Can you work these out from the model? Positions are in its coordinate system, mm. A direction names the side the tool comes from. Give positions to 0.01 mm unless a question says otherwise; leave off trailing zeros.
from build123d import *

# Parameters (mm, degrees)
BOSS_EXTRUDE2_DEPTH      = 52
FILLET2_R                = 1
CUT_EXTRUDE2_DEPTH       = 3
CUT_EXTRUDE2_DEPTH_BACK  = 6
SKETCH10_W               = 2.071027546
SKETCH10_H               = 17.5
SKETCH12_W               = 21
SKETCH12_H               = 29
BATTERY_DEPTH            = 0.4
SKETCH14_W               = 21.3
SKETCH14_H               = 1
BOSS_EXTRUDE4_DEPTH      = 7.999920354
FILLET5_R                = 1
SKETCH19_W               = 21.3
SKETCH19_H               = 1
BOSS_EXTRUDE5_DEPTH      = 2.6
SKETCH20_W               = 9.556221564
SKETCH20_H               = 2.6
CUT_EXTRUDE9_DEPTH       = 2.6
SKETCH21_W               = 21.3
SKETCH21_H               = 2.886084762
BOSS_EXTRUDE6_DEPTH      = 8
SKETCH23_W               = 24.481547991
SKETCH23_H               = 2.403526745
CUT_EXTRUDE10_DEPTH      = 2
SKETCH26_W               = 11.036128308
SKETCH26_H               = 2.126226966
CUT_EXTRUDE11_DEPTH      = 2
CUT_EXTRUDE12_DEPTH      = 2
CUT_EXTRUDE12_DEPTH_BACK = 11
SKETCH27_W               = 46
SKETCH27_H               = 2.33
CUT_EXTRUDE15_DEPTH      = 3
CUT_EXTRUDE15_DEPTH_BACK = 2
SKETCH30_W               = 16.027497941
SKETCH30_H               = 8.207966742
SKETCH32_W               = 21.3
SKETCH32_H               = 4.3
BOSS_EXTRUDE7_DEPTH      = 17
SKETCH33_W               = 15.5
SKETCH33_H               = 4.8
CUT_EXTRUDE16_DEPTH      = 17
CUT_EXTRUDE17_DEPTH      = 16
CUT_EXTRUDE17_DEPTH_BACK = 16
SKETCH34_W               = 15.546115034
SKETCH34_H               = 15
CHAMFER1_SIZE            = 2.050303842
CHAMFER1_SIZE_2          = 1
SKETCH36_W               = 1.919218309
SKETCH36_H               = 1.441495618
BOSS_EXTRUDE8_DEPTH      = 24
SKETCH37_W               = 15.546115034
SKETCH37_H               = 5.800639797
CUT_EXTRUDE18_DEPTH      = 3
SKETCH38_W               = 4.259754253
SKETCH38_H               = 3
BOSS_EXTRUDE9_DEPTH      = 7
FILLET6_R                = 2.5
BOSS_EXTRUDE10_DEPTH     = 18
SKETCH41_W               = 2.868853839
SKETCH41_H               = 1
SKETCH41_W_2             = 2.885031127
BOSS_EXTRUDE11_DEPTH     = 3
SKETCH42_W               = 6.004877842
SKETCH42_H               = 3.067097043
CUT_EXTRUDE19_DEPTH      = 7


with BuildPart() as part:
    # Sketch1 → Boss-Extrude2 (new body)
    with BuildSketch(Plane.XY):
        with BuildLine():
            Line((-4.570161627, 0), (-7.263800128, 0))
            add(Edge.make_bspline(
                [(0.042333709, 8.998333002), (-4.213116867, 8.648828695), (-5.985828681, 2.169241543), (-7.263800128, 0)],
                knots=[0, 0, 0, 0, 1, 1, 1, 1], degree=3))
            Line((0.042333709, 8.998333002), (0.742333709, 8.998333002))
            Line((0.742333709, 8.998333002), (0.742333709, 1))
            Line((0.742333709, 1), (22.042333709, 1))
            Line((22.042333709, 1), (22.042333709, 8.998333002))
            Line((22.042333709, 8.998333002), (23.042333709, 8.998333002))
            add(Edge.make_bspline(
                [(23.042333709, 8.998333002), (27.852391375, 8.27132168), (31.467788923, 0)],
                knots=[0, 0, 0, 1, 1, 1], degree=2))
            Line((31.467788923, 0), (26.875523276, 0))
            Line((26.875523276, 0), (22.86911945, 0))
            Line((22.86911945, 0), (0, 0))
            Line((0, 0), (-4.570161627, 0))
        make_face()
    extrude(amount=BOSS_EXTRUDE2_DEPTH)

    # Fillet2
    fillet2_edges = [part.edges().sort_by_distance(p)[0] for p in [
        (-7.263800128, 0, 26),
    ]]
    fillet(fillet2_edges, radius=FILLET2_R)

    # Sketch10 → Cut-Extrude2 (cut, two sides: drawn at the far end of the back side and taken through both)
    with BuildSketch(Plane(origin=(-4.432649633, 3.861619691, 0), x_dir=(0.6568701979277837, 0.7540036757697632, 0), z_dir=(-0.7540036757697632, 0.6568701979277837, 0)).offset(-CUT_EXTRUDE2_DEPTH_BACK)):
        with Locations((-0.442686988, -41.317163409)):
            Rectangle(SKETCH10_W, SKETCH10_H)
        with Locations((-0.442686988, -11.478878468)):
            Rectangle(SKETCH10_W, SKETCH10_H)
    extrude(amount=CUT_EXTRUDE2_DEPTH + CUT_EXTRUDE2_DEPTH_BACK, mode=Mode.SUBTRACT)

    # Sketch12 → Battery (cut)
    with BuildSketch(Plane(origin=(0, 1, 0), x_dir=(1, 0, 0), z_dir=(0, 1, 0))):
        with Locations((11.242333709, -36.5)):
            Rectangle(SKETCH12_W, SKETCH12_H)
    extrude(amount=-BATTERY_DEPTH, mode=Mode.SUBTRACT)

    # Sketch14 → Boss-Extrude4 (add)
    with BuildSketch(Plane(origin=(0, 1, 0), x_dir=(1, 0, 0), z_dir=(0, 1, 0))):
        with Locations((11.392333709, -51.5)):
            Rectangle(SKETCH14_W, SKETCH14_H)
    extrude(amount=BOSS_EXTRUDE4_DEPTH)

    # Fillet5
    fillet5_edges = [part.edges().sort_by_distance(p)[0] for p in [
        (31.467788923, 0, 26),
    ]]
    fillet(fillet5_edges, radius=FILLET5_R)

    # Sketch19 → Boss-Extrude5 (add)
    with BuildSketch(Plane(origin=(0, 0, 51), x_dir=(-1, 0, 0), z_dir=(0, 0, -1))):
        with Locations((-11.392333709, 5)):
            Rectangle(SKETCH19_W, SKETCH19_H)
    extrude(amount=BOSS_EXTRUDE5_DEPTH)

    # Sketch20 → Cut-Extrude9 (cut)
    with BuildSketch(Plane(origin=(0, 5.5, 0), x_dir=(1, 0, 0), z_dir=(0, 1, 0))):
        with Locations((10.971722634, -49.7)):
            Rectangle(SKETCH20_W, SKETCH20_H)
    extrude(amount=-CUT_EXTRUDE9_DEPTH, mode=Mode.SUBTRACT)

    # Sketch21 → Boss-Extrude6 (add)
    with BuildSketch(Plane(origin=(0, 1, 0), x_dir=(1, 0, 0), z_dir=(0, 1, 0))):
        with Locations((11.392333709, -18.443042381)):
            Rectangle(SKETCH21_W, SKETCH21_H)
    extrude(amount=BOSS_EXTRUDE6_DEPTH)

    # Sketch23 → Cut-Extrude10 (cut)
    with BuildSketch(Plane(origin=(0.742333709, 0, 0), x_dir=(0, 0, -1), z_dir=(1, 0, 0))):
        with Locations((-32.126858758, 6.701763373)):
            Rectangle(SKETCH23_W, SKETCH23_H)
    extrude(amount=-CUT_EXTRUDE10_DEPTH, mode=Mode.SUBTRACT)

    # Sketch26 → Cut-Extrude11 (cut)
    with BuildSketch(Plane(origin=(0, 0, 51), x_dir=(-1, 0, 0), z_dir=(0, 0, -1))):
        with Locations((-6.260397863, 7.936806871)):
            Rectangle(SKETCH26_W, SKETCH26_H)
    extrude(amount=-CUT_EXTRUDE11_DEPTH, mode=Mode.SUBTRACT)

    # Sketch27 → Cut-Extrude12 (cut, two sides: drawn at the far end of the back side and taken through both)
    with BuildSketch(Plane(origin=(15.71645511, 16.134429341, 0), x_dir=(0, 0, -1), z_dir=(0.6977674498915984, 0.7163243580053493, 0)).offset(-CUT_EXTRUDE12_DEPTH_BACK)):
        with Locations((-26, -18.013212029)):
            Rectangle(SKETCH27_W, SKETCH27_H)
    extrude(amount=CUT_EXTRUDE12_DEPTH + CUT_EXTRUDE12_DEPTH_BACK, mode=Mode.SUBTRACT)

    # Sketch30 → Cut-Extrude15 (cut, two sides: drawn at the far end of the back side and taken through both)
    with BuildSketch(Plane(origin=(-4.432649633, 3.861619691, 0), x_dir=(0.6568701979277837, 0.7540036757697632, 0), z_dir=(-0.7540036757697632, 0.6568701979277837, 0)).offset(-CUT_EXTRUDE15_DEPTH_BACK)):
        with Locations((1.087669114, -26.408883952)):
            Rectangle(SKETCH30_W, SKETCH30_H)
    extrude(amount=CUT_EXTRUDE15_DEPTH + CUT_EXTRUDE15_DEPTH_BACK, mode=Mode.SUBTRACT)

    # Sketch32 → Boss-Extrude7 (add)
    with BuildSketch(Plane(origin=(0, 0, 0), x_dir=(-1, 0, 0), z_dir=(0, 0, -1))):
        with Locations((-11.392333709, 3.15)):
            Rectangle(SKETCH32_W, SKETCH32_H)
    extrude(amount=-BOSS_EXTRUDE7_DEPTH)

    # Sketch33 → Cut-Extrude16 (cut)
    with BuildSketch(Plane(origin=(0, 0, 0), x_dir=(-1, 0, 0), z_dir=(0, 0, -1))):
        with Locations((-11.42347987, 2.9)):
            Rectangle(SKETCH33_W, SKETCH33_H)
    extrude(amount=-CUT_EXTRUDE16_DEPTH, mode=Mode.SUBTRACT)

    # Sketch34 → Cut-Extrude17 (cut, two sides: drawn at the far end of the back side and taken through both)
    with BuildSketch(Plane(origin=(0, 0.5, 0), x_dir=(1, 0, 0), z_dir=(0, 1, 0)).offset(-CUT_EXTRUDE17_DEPTH_BACK)):
        with Locations((11.400422353, -9.617701537)):
            Rectangle(SKETCH34_W, SKETCH34_H)
    extrude(amount=CUT_EXTRUDE17_DEPTH + CUT_EXTRUDE17_DEPTH_BACK, mode=Mode.SUBTRACT)

    # Chamfer1
    # the kernel refuses this chamfer: 2.050303842, 1 mm, written as the material it takes off along each edge
    with BuildSketch(Plane(origin=(19.17347987, 0.5, 2.117701537), x_dir=(0, 0.016923890849829, -0.9998567807033681), z_dir=(-1, 0, 0))) as chamfer1_piece_1:
        Polygon((CHAMFER1_SIZE * 0.999856780498, CHAMFER1_SIZE * 0.0169238908464), (-CHAMFER1_SIZE_2 * 0.0169238908498, CHAMFER1_SIZE_2 * 0.999856780703), (0, 0), align=None)
    extrude(amount=15.5, mode=Mode.SUBTRACT)

    # Sketch36 → Boss-Extrude8 (add)
    with BuildSketch(Plane(origin=(0.742333709, 0, 0), x_dir=(0, 0, -1), z_dir=(1, 0, 0))):
        with Locations((-0.959609155, 6.020747809)):
            Rectangle(SKETCH36_W, SKETCH36_H)
    extrude(amount=BOSS_EXTRUDE8_DEPTH)

    # Sketch37 → Cut-Extrude18 (cut)
    with BuildSketch(Plane(origin=(0, 0, 17.117701537), x_dir=(-1, 0, 0), z_dir=(0, 0, -1))):
        with Locations((-11.400422353, 4.08463089)):
            Rectangle(SKETCH37_W, SKETCH37_H)
    extrude(amount=-CUT_EXTRUDE18_DEPTH, mode=Mode.SUBTRACT)

    # Sketch38 → Boss-Extrude9 (add)
    with BuildSketch(Plane(origin=(0, 1.184310992, 0), x_dir=(1, 0, 0), z_dir=(0, 1, 0))):
        with Locations((11.677903031, -18.617701537)):
            Rectangle(SKETCH38_W, SKETCH38_H)
    extrude(amount=BOSS_EXTRUDE9_DEPTH)

    # Fillet6
    # the kernel refuses this fillet: 2.5 mm, written as the material it takes off along each edge
    with BuildSketch(Plane(origin=(14.862488739, 1.184310992, 17.117701537), x_dir=(0, -1, 0), z_dir=(-1, 0, 0))) as fillet6_piece_1_section:
        with BuildLine():
            CenterArc((2.5, 2.125785134), FILLET6_R, 180, 58.245844015)
            Line((0, 2.125785134), (-0.05, 2.125785134))
            Line((-0.05, 2.125785134), (-0.05, 0))
            Line((-0.05, 0), (0, -0.05))
            ThreePointArc((0, -0.05), (0.592155496, -0.05), (1.157997212, -0.042515703))
            Line((1.157997212, -0.042515703), (1.184310992, 0))
        make_face()
    fillet6_piece_1 = extrude(amount=11.235123902, mode=Mode.PRIVATE)
    fillet6_piece_1 = split(fillet6_piece_1, bisect_by=Plane(origin=(13.807780157, 0.878026012, 17.652561739), z_dir=(1, 0, 0)), keep=Keep.TOP, mode=Mode.PRIVATE)
    add(fillet6_piece_1, mode=Mode.SUBTRACT)
    with BuildSketch(Plane(origin=(9.548025904, 1.184310992, 17.117701537), x_dir=(0, -1, 0), z_dir=(-1, 0, 0))) as fillet6_piece_2:
        with BuildLine():
            CenterArc((2.5, 2.125785134), FILLET6_R, 180, 58.245844015)
            Line((0, 2.125785134), (-0.05, 2.125785134))
            Line((-0.05, 2.125785134), (-0.05, 0))
            Line((-0.05, 0), (0, -0.05))
            ThreePointArc((0, -0.05), (0.592155496, -0.05), (1.157997212, -0.042515703))
            Line((1.157997212, -0.042515703), (1.184310992, 0))
        make_face()
    extrude(amount=5.920661068, mode=Mode.SUBTRACT)
    with BuildSketch(Plane(origin=(19.17347987, 1.184310992, 17.117701537), x_dir=(0, -1, 0), z_dir=(-1, 0, 0))) as fillet6_piece_3:
        with BuildLine():
            CenterArc((2.5, 2.125785134), FILLET6_R, 180, 58.245844015)
            Line((0, 2.125785134), (-0.05, 2.125785134))
            Line((-0.05, 2.125785134), (-0.05, 0))
            Line((-0.05, 0), (0, -0.05))
            ThreePointArc((0, -0.05), (0.592155496, -0.05), (1.157997212, -0.042515703))
            Line((1.157997212, -0.042515703), (1.184310992, 0))
        make_face()
    extrude(amount=5.365699713, mode=Mode.SUBTRACT)
    with BuildSketch(Plane(origin=(19.17347987, 1.184310992, 17.117701537), x_dir=(0, -1, 0), z_dir=(-1, 0, 0))) as fillet6_piece_4_section:
        with BuildLine():
            CenterArc((2.5, 2.125785134), FILLET6_R, 180, 58.245844015)
            Line((0, 2.125785134), (-0.05, 2.125785134))
            Line((-0.05, 2.125785134), (-0.05, 0))
            Line((-0.05, 0), (0, -0.05))
            ThreePointArc((0, -0.05), (0.592155496, -0.05), (1.157997212, -0.042515703))
            Line((1.157997212, -0.042515703), (1.184310992, 0))
        make_face()
    fillet6_piece_4 = extrude(amount=10.680162547, mode=Mode.PRIVATE)
    fillet6_piece_4 = split(fillet6_piece_4, bisect_by=Plane(origin=(9.548025904, 0.878026012, 17.652561739), z_dir=(-1, 0, 0)), keep=Keep.TOP, mode=Mode.PRIVATE)
    add(fillet6_piece_4, mode=Mode.SUBTRACT)

    # Sketch40 → Boss-Extrude10 (add)
    with BuildSketch(Plane(origin=(3.67347987, 0, 0), x_dir=(0, 0, -1), z_dir=(1, 0, 0))):
        Polygon((-1.194674299, 0), (-2.117701537, 0), (-2.117701537, 0.29858263), (-1.194674299, 0.29858263), (-0.66544558, 0.29858263), (-0.66544558, 0), align=None)
    extrude(amount=BOSS_EXTRUDE10_DEPTH)

    # Sketch41 → Boss-Extrude11 (add)
    with BuildSketch(Plane.XY.offset(19.886084762)):
        with Locations((20.607906789, 5)):
            Rectangle(SKETCH41_W, SKETCH41_H)
        with Locations((2.184849273, 5)):
            Rectangle(SKETCH41_W_2, SKETCH41_H)
    extrude(amount=BOSS_EXTRUDE11_DEPTH)

    # Sketch42 → Cut-Extrude19 (cut)
    with BuildSketch(Plane(origin=(0, 9, 0), x_dir=(1, 0, 0), z_dir=(0, 1, 0))):
        with Locations((11.52664117, -19.791450538)):
            Rectangle(SKETCH42_W, SKETCH42_H)
    extrude(amount=-CUT_EXTRUDE19_DEPTH, mode=Mode.SUBTRACT)


solid = part.part
(1) Thinking about a two-plate mould opening in X: for faces 1 (the flat face through (-2.782, 2.712, 26.351)), 2 (the flat face through (0.742, 4, 39)), 3 (the flat face through (11, 9, 18)), which applies, pulls with the +X half, pulls with the -X half, needs draft (parallel to the pull), parting line crosses it, or undercut?
Returned:
face 1: pulls with the -X half
face 2: undercut
face 3: needs draft
(2) Please list where these lines run through material, in increasing order: probe 1 along Z at (x, y) = (21.5, 7.25); probe 2 along Z at (x, y) = (19, 8.75); probe 3 along Z at (x, y) = (-4, 3.5).
Returned:
probe 1: z = 17 to 19.89, 51 to 52
probe 2: z = 17.12 to 19.89, 51 to 52
probe 3: z = 0 to 2.73, 20.23 to 22.3, 30.51 to 32.57, 50.07 to 52
(3) Will these pins go through, and if not, where does the flat tip stop? P1, Ø4, axis at x = 20.5, z = 33, coming from the +Y side; P2, Ø4, axis at x = 11.5, y = 3, coming from the -Z side; P3, Ø1.5, axis at y = 5.5, z = 9.5, coming from the +X side; P4, Ø0.9, axis at x = 20.5, z = 21.5, coming from the +Y side.
Returned:
P1: stops at y = 9
P2: stops at z = 17.12
P3: stops at x = 28.56
P4: stops at y = 5.5
(4) Suppose I cut it at A-A on x = 18.5. Give the number of separate pieces and of enclosed holes in the cut face, plus the area to 3 significant figures.
Returned:
separate pieces: 4
enclosed holes: 0
area: 42.7 mm2
(5) Which directions (+Z, -Z, +X, -X, +Y, -Y) give clear straight access to the entire face, cutting with the end or side of a thin tool? Please do faces 4 (the flat face through (19, 4.5, 50)), 5 (the flat face through (21, 5, 22.886)), 6 (the flat face through (8.524, 8, 19)).
Returned:
face 4: none
face 5: +Y
face 6: +Z, +Y
